For this review, take the finished solid that the model builds, in its own axes (mm). Round coordinates to 2 decimals unless told otherwise and drop trailing zeros. Order: outer loops, then holes, each group sorted by start corner. A loop starts at its lowest first (then second) coordinate and runs counter-clockwise, first axis right, second up. Notation, with made-up numbers: M 16.25,33.5 L 52.25,33.5 A8 ccw 52.25,44.5 Z; hole C 56,1.5 d1. An arc over 180 degrees is marked long. Use a Markdown table: item, result.
from build123d import *

# Parameters (mm, degrees)
SKETCH1_W           = 75
SKETCH1_H           = 25
BOSS_EXTRUDE1_DEPTH = 2.5
SKETCH2_W           = 1.5
SKETCH2_H           = 4
SKETCH2_H_2         = 2.5
SKETCH2_H_3         = 4.75
CUT_EXTRUDE1_DEPTH  = 1


with BuildPart() as part:
    # Sketch1 → Boss-Extrude1 (new body)
    with BuildSketch(Plane(origin=(0, 0, 0), x_dir=(1, 0, 0), z_dir=(0, 1, 0))):
        Rectangle(SKETCH1_W, SKETCH1_H)
    extrude(amount=BOSS_EXTRUDE1_DEPTH)

    # Sketch2 → Cut-Extrude1 (cut)
    with BuildSketch(Plane(origin=(0, 2.5, 0), x_dir=(1, 0, 0), z_dir=(0, 1, 0))):
        Polygon((6, 1.5), (6, -1.5), (7.5, -1.5), (14.5, -1.5), (16, -1.5), (16, -1), (16, 0), (16, 1.5), (14.5, 1.5), align=None)
        with Locations((6.75, -3.5)):
            Rectangle(SKETCH2_W, SKETCH2_H)
        with Locations((15.25, -2.75)):
            Rectangle(SKETCH2_W, SKETCH2_H_2)
        with Locations((15.25, 2.75)):
            Rectangle(SKETCH2_W, SKETCH2_H_2)
        Polygon((16, -4), (14.5, -4), (14.5, -5.5), (19, -5.5), (19, -4), align=None)
        Polygon((14.5, 5.5), (14.5, 4), (16, 4), (21, 4), (22.5, 4), (22.5, 5.5), align=None)
        with Locations((21.75, 1.625)):
            Rectangle(SKETCH2_W, SKETCH2_H_3)
        Polygon((-16.5, 1.5), (-16.5, -1.5), (-15, -1.5), (-8, -1.5), (-6.5, -1.5), (-6.5, -1), (-6.5, 0), (-6.5, 1.5), (-8, 1.5), align=None)
        with Locations((-15.75, -3.5)):
            Rectangle(SKETCH2_W, SKETCH2_H)
        with Locations((-7.25, -2.75)):
            Rectangle(SKETCH2_W, SKETCH2_H_2)
        with Locations((-7.25, 2.75)):
            Rectangle(SKETCH2_W, SKETCH2_H_2)
        Polygon((-6.5, -4), (-8, -4), (-8, -5.5), (-3.5, -5.5), (-3.5, -4), align=None)
        Polygon((-8, 5.5), (-8, 4), (-6.5, 4), (-1.5, 4), (0, 4), (0, 5.5), align=None)
        with Locations((-0.75, 1.625)):
            Rectangle(SKETCH2_W, SKETCH2_H_3)
    extrude(amount=-CUT_EXTRUDE1_DEPTH, mode=Mode.SUBTRACT)


solid = part.part
Q1. Draft analysis for pull direction Z (two halves, no side actions). For faces 1 (the flat face through (-1, 1, 12.5)), 2 (the flat face through (-37.5, 1, 0)), 3 (the flat face through (-8, 1.5, 0)), state which applies: pulls with the +Z half, pulls with the -Z half, needs draft (parallel to the pull), parting line crosses it, or undercut.
Determined:
| item | result |
|---|---|
| face 1 | pulls with the +Z half |
| face 2 | needs draft |
| face 3 | undercut |
Q2. Add section B-B (z = -2.75). Write out the cut boundary in (x, y).
Determined:
| item | result |
|---|---|
| outline | M -37.5,0 L 37.5,0 L 37.5,2.5 L 22.5,2.5 L 22.5,1.5 L 21,1.5 L 21,2.5 L 16,2.5 L 16,1.5 L 14.5,1.5 L 14.5,2.5 L 0,2.5 L 0,1.5 L -1.5,1.5 L -1.5,2.5 L -6.5,2.5 L -6.5,1.5 L -8,1.5 L -8,2.5 L -37.5,2.5 Z |
Q3. Wall thickness on line 1 along X through (y, z) = (2.15, -2.5); line 2 along Z through (x, y) = (-13.5, 1.85); line 3 along Z through (x, y) = (20, 2.15): over which ranges is each line inside the solid? List them lowest first. Write a range as [from, to].
Determined:
| item | result |
|---|---|
| line 1 | x = [-37.5, -8], [-6.5, -1.5], [0, 14.5], [16, 21], [22.5, 37.5] |
| line 2 | z = [-12.5, -1.5], [1.5, 12.5] |
| line 3 | z = [-12.5, -5.5], [-4, 12.5] |
Q4. Add section A-A (x = -12). Write out the cut boundary in (y, z), then the cut area to 3 significant figures.
Determined:
| item | result |
|---|---|
| outline | M 0,-12.5 L 2.5,-12.5 L 2.5,-1.5 L 1.5,-1.5 L 1.5,1.5 L 2.5,1.5 L 2.5,12.5 L 0,12.5 Z |
| area | 59.5 mm^2 |
